The listing builds one solid part. Answer for the finished solid, in the listing's coordinates (mm). A direction names the side the tool comes from. Coordinates: 2 decimals unless noted, no trailing zeros. Loops run counter-clockwise (first coordinate to the right, second up) from the corner with the lowest first, then second, coordinate; pieces in that order, holes last. Notation, with made-up numbers: (73, -7.75) -> (99, -7.75) arc R17 ccw to (99, 8.25) -> close; hole circle Ø6 at (-14.5, 16.5). An arc over 180 degrees is marked (long way). Answer in a Markdown table with one row per item.
```python
from build123d import *

# Parameters (mm, degrees)
ESQUISSE1_R        = 2.2
BOSS_EXTRU_1_DEPTH = 1.85
ESQUISSE2_R        = 1.25
BOSS_EXTRU_2_DEPTH = 12.05
CHANFREIN1_SIZE    = 1.85
CHANFREIN1_SIZE_2  = 0.3
CONG_1_R           = 0.1


with BuildPart() as part:
    # Esquisse1 → Boss.-Extru.1 (new body)
    with BuildSketch(Plane(origin=(0, 0, 0), x_dir=(1, 0, 0), z_dir=(0, 1, 0))):
        with Locations(Location((0, 0, 0), (0, 0, 270))):
            Circle(ESQUISSE1_R)
    extrude(amount=BOSS_EXTRU_1_DEPTH)

    # Esquisse2 → Boss.-Extru.2 (add)
    with BuildSketch(Plane(origin=(0, 1.85, 0), x_dir=(1, 0, 0), z_dir=(0, 1, 0))):
        with Locations(Location((0, 0, 0), (0, 0, 270))):
            Circle(ESQUISSE2_R)
    extrude(amount=BOSS_EXTRU_2_DEPTH)

    # Chanfrein1
    # the kernel refuses this chamfer: 1.85, 0.3 mm, written as the material it takes off along each edge
    with BuildSketch(Plane(origin=(0, 0, 0), x_dir=(0, 0, 1), z_dir=(-1, 0, 0))) as chanfrein1_piece_1:
        Polygon((2.2, CHANFREIN1_SIZE), (2.2 - CHANFREIN1_SIZE_2, 0), (2.2, 0), align=None)
    revolve(axis=Axis((0, 0, 0), (0, 1, 0)), mode=Mode.SUBTRACT)

    # Congé1
    cong_1_edges = [part.edges().sort_by_distance(p)[0] for p in [
        (0, 0, -1.9),
    ]]
    fillet(cong_1_edges, radius=CONG_1_R)


solid = part.part
```
Item 1: Flat-ended cylindrical pins translate along their axes: pin 1 Ø1.5 at (x, y) = (-0.5, 6) entering from -Z; pin 2 Ø1 at (x, y) = (-1.5, 10.5) entering from -Z. Find the tip coordinate at first contact, or state that the pin passes through.
Findings below:
| item | result |
|---|---|
| pin 1 | stops at z = -1.25 |
| pin 2 | stops at z = -0.75 |
Item 2: A cutting plane is placed at A-A, the plane z = 0. Determine the outline of the cut face in (x, y).
Findings below:
| item | result |
|---|---|
| outline | (-2.2, 1.85) -> (-1.91, 0.08) arc R0.1 ccw to (-1.81, 0) -> (1.81, 0) arc R0.1 ccw to (1.91, 0.08) -> (2.2, 1.85) -> (1.25, 1.85) -> (1.25, 13.9) -> (-1.25, 13.9) -> (-1.25, 1.85) -> close |
Item 3: A cutting plane is placed at B-B, the plane x = 0. Determine the outline of the cut face in (y, z).
Findings below:
| item | result |
|---|---|
| outline | (0, -1.81) arc R0.1 ccw to (0.08, -1.91) -> (1.85, -2.2) -> (1.85, -1.25) -> (13.9, -1.25) -> (13.9, 1.25) -> (1.85, 1.25) -> (1.85, 2.2) -> (0.08, 1.91) arc R0.1 ccw to (0, 1.81) -> close |
Item 4: A cutting plane is placed at C-C, the plane y = 11.5. Determine the outline of the cut face in (x, z), plus the area to 3 significant figures.
Findings below:
| item | result |
|---|---|
| outline | circle Ø2.5 at (0, 0) |
| area | 4.91 mm2 |
Item 5: Find the intervals of material crossed by probe 1 along Y at (x, z) = (-1.5, 0.2); probe 2 along X at (y, z) = (0.75, -1.05); probe 3 along X at (y, z) = (9, 0.55), in increasing order.
Findings below:
| item | result |
|---|---|
| probe 1 | y = 0 to 1.85 |
| probe 2 | x = -1.73 to 1.73 |
| probe 3 | x = -1.12 to 1.12 |
Item 6: A tool of negligible diameter and unlimited length cuts with its end or side. For faces 1 (the face through (0, 0, 0)), 2 (the face through (-1.22, 7.79, -0.27)), from which of +Z, -Z, +X, -X, +Y, -Y can it reach the whole face along a straight path? Write none if from no direction.
Findings below:
| item | result |
|---|---|
| face 1 | +Z, -Z, +X, -X, -Y |
| face 2 | +Y |
